from build123d import *

# Parameters (mm, degrees)
ESQUISSE2_R                  = 0.6
ENL_V_MAT_EXTRU_1_DEPTH      = 3
ENL_V_MAT_EXTRU_1_DEPTH_BACK = 3


with BuildPart() as part:
    # Esquisse1 → Révolution1 (revolve)
    with BuildSketch(Plane(origin=(0, 0, 0), x_dir=(0, 0, -1), z_dir=(1, 0, 0))):
        Polygon((-5.5, 0), (-5.5, 1), (-0.5, 1), (-0.5, 2), (5.5, 2), (5.5, 1.5), (1.5, 1.5), (1.5, 0), align=None)
    revolve(axis=Axis((0, 0, 5.5), (0, 0, -1)))

    # Esquisse2 → Enlèv. mat.-Extru.1 (cut, two sides)
    with BuildSketch(Plane(origin=(0, 0, 0), x_dir=(1, 0, 0), z_dir=(0, 1, 0))) as enl_v_mat_extru_1_sk:
        with Locations((0, 2.5)):
            Circle(ESQUISSE2_R)
    extrude(amount=ENL_V_MAT_EXTRU_1_DEPTH, mode=Mode.SUBTRACT)
    extrude(enl_v_mat_extru_1_sk.sketch, amount=-ENL_V_MAT_EXTRU_1_DEPTH_BACK, mode=Mode.SUBTRACT)


solid = part.part
Build history of the part. All positions in model axes, mm. A direction names the side the tool comes from. Round coordinates to 2 decimals unless told otherwise and drop trailing zeros. Loops run counter-clockwise (first coordinate to the right, second up) from the corner with the lowest first, then second, coordinate; pieces in that order, holes last. Notation, with made-up numbers: (42.25, 68) -> (49.25, 68) arc R8 ccw to (49.25, 77) -> close; hole circle Ø1 at (-1, 89). An arc over 180 degrees is marked (long way). One line per item, written item: value. Start each with the question number.
Q1. Cut at D-D on x = -1.2. List the corners of the cut face in (y, z), plus the area to 3 significant figures.
Q2. Cut at A-A on x = 0. List the corners of the cut face in (y, z).
Q3. Probe line 1 along X through (y, z) = (0, -2.6); line 2 along Z through (x, y) = (0, 1.85). List the from-to ranges inside material, lowest first.
Q4. Two-plate mould, pull along X, no slides. Class faces 1 (the face through (0, 0, -1.5)), 2 (the face through (0, 0, 5.5)), 3 (the face through (-1, 0, 3)): released by +X, released by -X, zero draft, split by the parting line, or undercut.
Q5. Drop a flat-ended pin along its axis: pin 1 Ø1.5 at (y, z) = (1, 0.5) entering from -X. Give the stop position or say it passes through.
Q6. Cut at B-B on z = -2.5. List the corners of the cut face in (x, y), plus the area to 3 significant figures.
Q7. Cut at C-C on y = -0.3. List the corners of the cut face in (x, z).
Q8. 3-axis set-ups, long thin cutter, end or side, ignore diameter. For faces 4 (the face through (0.572, 1.683, -2.68)), 5 (the face through (-1, -1, 0.5)), 6 (the face through (-1.33, 0.69, -3.47)): which of +Z, -Z, +X, -X, +Y, -Y reach the whole face in a straight line?
Computed:
1. outline: (-1.6, -5.5) -> (-0.9, -5.5) -> (-0.9, -1.5) -> (0.9, -1.5) -> (0.9, -5.5) -> (1.6, -5.5) -> (1.6, 0.5) -> (-1.6, 0.5) -> close
1. area: 12.0 mm²
2. outline: (-2, -5.5) -> (-1.5, -5.5) -> (-1.5, -3.1) -> (-2, -3.1) -> close; (-2, -1.9) -> (-1.5, -1.9) -> (-1.5, -1.5) -> (1.5, -1.5) -> (1.5, -1.9) -> (2, -1.9) -> (2, 0.5) -> (1, 0.5) -> (1, 5.5) -> (-1, 5.5) -> (-1, 0.5) -> (-2, 0.5) -> close; (1.5, -5.5) -> (2, -5.5) -> (2, -3.1) -> (1.5, -3.1) -> close
3. line 1: -2 to -1.5, 1.5 to 2
3. line 2: -5.5 to -3.1, -1.9 to 0.5
4. face 1: undercut
4. face 2: zero draft
4. face 3: split by the parting line
5. pin 1: x = -1.98
6. outline: (-0.6, -1.91) -> (-0.6, -1.37) arc R1.5 cw to (-0.6, 1.37) -> (-0.6, 1.91) arc R2 ccw to start; (0.6, -1.91) arc R2 ccw to (0.6, 1.91) -> (0.6, 1.37) arc R1.5 cw to (0.6, -1.37) -> close
6. area: 4.27 mm²
7. outline: (-1.98, -5.5) -> (-1.47, -5.5) -> (-1.47, -1.5) -> (1.47, -1.5) -> (1.47, -5.5) -> (1.98, -5.5) -> (1.98, 0.5) -> (0.95, 0.5) -> (0.95, 5.5) -> (-0.95, 5.5) -> (-0.95, 0.5) -> (-1.98, 0.5) -> close
8. face 4: +Y, -Y
8. face 5: +Z
8. face 6: -Z
